For this review, use the dimensioned drawing (mm, ordinates from the lowest corner) and the shaded views. Round coordinates to 2 decimals unless told otherwise and drop trailing zeros. Loops run counter-clockwise (first coordinate to the right, second up) from the corner with the lowest first, then second, coordinate; pieces in that order, holes last. Notation, with made-up numbers: (41.5, -9) -> (65.5, -9) arc R29 ccw to (65.5, 25) -> close; hole circle Ø3 at (31.25, 87.5). An arc over 180 degrees is marked (long way). Write each question's results on one line, items separated by ' | '.
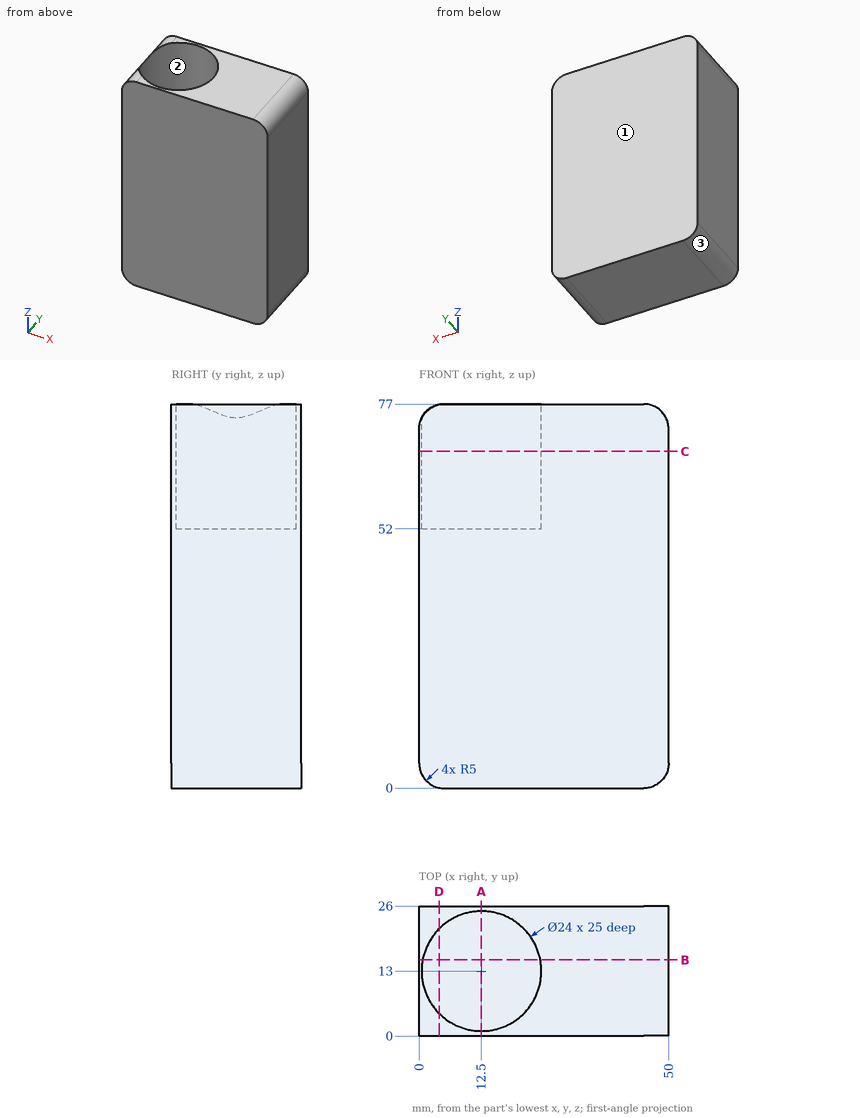
1. Draft analysis for pull direction Y (two halves, no side actions). For the marked faces 1, 2 and 3, state which applies: released by +Y, released by -Y, zero draft, split by the parting line, or undercut.
Values found:
face 1: released by +Y | face 2: undercut | face 3: zero draft
2. Consider section D-D (x = 4). State the section outline as (y, z) points, plus the area to 3 significant figures.
Values found:
outline: (0, 0.1) -> (26, 0.1) -> (26, 76.9) -> (21.47, 76.9) -> (21.47, 52) -> (4.53, 52) -> (4.53, 76.9) -> (0, 76.9) -> close | area: 1,570 mm2
3. Consider section B-B (y = 15.25). State the section outline as (x, z) points.
Values found:
outline: (0, 5) arc R5 ccw to (5, 0) -> (45, 0) arc R5 ccw to (50, 5) -> (50, 72) arc R5 ccw to (45, 77) -> (24.29, 77) -> (24.29, 52) -> (0.71, 52) -> (0.71, 74.57) arc R5 ccw to (0, 72) -> close
4. Consider section C-C (z = 67.5). State the section outline as (x, y) points.
Values found:
outline: (0, 0) -> (50, 0) -> (50, 26) -> (0, 26) -> close; hole circle Ø24 at (12.5, 13)
5. Consider section A-A (x = 12.5). State the section outline as (y, z) points, plus the area to 3 significant figures.
Values found:
outline: (0, 0) -> (26, 0) -> (26, 77) -> (25, 77) -> (25, 52) -> (1, 52) -> (1, 77) -> (0, 77) -> close | area: 1,400 mm2
6. For pin 1 (8 mm diameter, centred on x = 39.5, y = 19, fed in from -Z), flat-tipped, find the tip position at first contact; note if it passes through.
Values found:
pin 1: stops at z = 0
7. To check wall thickness, follow probe 1 along X at (y, z) = (13, 67); probe 2 along Y at (x, z) = (12.5, 66.5); probe 3 along Y at (x, z) = (22, 61.5). State the ranges of each line that lie inside material, in increasing order.
Values found:
probe 1: x = 0 to 0.5, 24.5 to 50 | probe 2: y = 0 to 1, 25 to 26 | probe 3: y = 0 to 5.67, 20.33 to 26
